```python
from build123d import *

# Parameters (mm, degrees)
BOSS_EXTRUDE1_DEPTH = 12
BOSS_EXTRUDE2_DEPTH = 4.5
FILLET1_R           = 5
FILLET2_R           = 1.5
CUT_EXTRUDE1_DEPTH  = 1
CUT_EXTRUDE2_DEPTH  = 1.5
CUT_EXTRUDE3_DEPTH  = 0.5
FILLET3_R           = 1.5


with BuildPart() as part:
    # Sketch1 → Boss-Extrude1 (new body)
    with BuildSketch(Plane(origin=(0, 0, 0), x_dir=(1, 0, 0), z_dir=(0, 1, 0))):
        with BuildLine():
            Line((-149.337, -110.617), (149.337, -110.617))
            ThreePointArc((149.337, -110.617), (154.286747468, -108.566747468), (156.337, -103.617))
            Line((156.337, -103.617), (156.337, 103.617))
            ThreePointArc((156.337, 103.617), (154.286747468, 108.566747468), (149.337, 110.617))
            Line((149.337, 110.617), (-149.337, 110.617))
            ThreePointArc((-149.337, 110.617), (-154.286747468, 108.566747468), (-156.337, 103.617))
            Line((-156.337, 103.617), (-156.337, -103.617))
            ThreePointArc((-156.337, -103.617), (-154.286747468, -108.566747468), (-149.337, -110.617))
        make_face()
    extrude(amount=BOSS_EXTRUDE1_DEPTH)

    # Sketch2 → Boss-Extrude2 (add)
    with BuildSketch(Plane(origin=(0, 0, -110.617), x_dir=(-1, 0, 0), z_dir=(0, 0, -1))):
        with BuildLine():
            Line((-149.337, 6), (149.337, 6))
            ThreePointArc((149.337, 6), (154.286747468, 8.050252532), (156.337, 13))
            Line((156.337, 13), (156.337, 221))
            ThreePointArc((156.337, 221), (154.286747468, 225.949747468), (149.337, 228))
            Line((149.337, 228), (-149.337, 228))
            ThreePointArc((-149.337, 228), (-154.286747468, 225.949747468), (-156.337, 221))
            Line((-156.337, 221), (-156.337, 13))
            ThreePointArc((-156.337, 13), (-154.286747468, 8.050252532), (-149.337, 6))
        make_face()
    extrude(amount=BOSS_EXTRUDE2_DEPTH)

    # Fillet1
    fillet1_edges = [part.edges().sort_by_distance(p)[0] for p in [
        (-156.337, 0, 0),
        (-154.286747468, 0, -108.566747468),
        (0, 0, -110.617),
        (154.286747468, 0, -108.566747468),
        (156.337, 0, 0),
        (154.286747468, 0, 108.566747468),
        (0, 0, 110.617),
        (-154.286747468, 0, 108.566747468),
    ]]
    fillet(fillet1_edges, radius=FILLET1_R)

    # Fillet2
    fillet2_edges = [part.edges().sort_by_distance(p)[0] for p in [
        (154.286747468, 8.050252532, -115.117),
        (0, 6, -115.117),
        (-154.286747468, 8.050252532, -115.117),
        (-156.337, 117, -115.117),
        (-154.286747468, 225.949747468, -115.117),
        (0, 228, -115.117),
        (154.286747468, 225.949747468, -115.117),
        (156.337, 117, -115.117),
    ]]
    fillet(fillet2_edges, radius=FILLET2_R)

    # Sketch3 → Cut-Extrude1 (cut)
    with BuildSketch(Plane.XY.offset(-110.617)):
        with BuildLine():
            Line((-151.337, 8.417424305), (151.337, 8.417424305))
            ThreePointArc((151.337, 8.417424305), (153.520300133, 10.261387212), (154.337, 13))
            Line((154.337, 13), (154.337, 221))
            ThreePointArc((154.337, 221), (152.872533906, 224.535533906), (149.337, 226))
            Line((149.337, 226), (-149.337, 226))
            ThreePointArc((-149.337, 226), (-152.872533906, 224.535533906), (-154.337, 221))
            Line((-154.337, 221), (-154.337, 13))
            ThreePointArc((-154.337, 13), (-153.520300133, 10.261387212), (-151.337, 8.417424305))
        make_face()
    extrude(amount=-CUT_EXTRUDE1_DEPTH, mode=Mode.SUBTRACT)

    # Sketch4 → Cut-Extrude2 (cut)
    with BuildSketch(Plane(origin=(0, 12, 0), x_dir=(1, 0, 0), z_dir=(0, 1, 0))):
        with BuildLine():
            Line((-134.337, -20.617), (134.337, -20.617))
            ThreePointArc((134.337, -20.617), (137.872533906, -19.152533906), (139.337, -15.617))
            Line((139.337, -15.617), (139.337, 88.617))
            ThreePointArc((139.337, 88.617), (137.872533906, 92.152533906), (134.337, 93.617))
            Line((134.337, 93.617), (-134.337, 93.617))
            ThreePointArc((-134.337, 93.617), (-137.872533906, 92.152533906), (-139.337, 88.617))
            Line((-139.337, 88.617), (-139.337, -15.617))
            ThreePointArc((-139.337, -15.617), (-137.872533906, -19.152533906), (-134.337, -20.617))
        make_face()
    extrude(amount=-CUT_EXTRUDE2_DEPTH, mode=Mode.SUBTRACT)

    # Sketch4<3> → Cut-Extrude3 (cut)
    with BuildSketch(Plane(origin=(0, 12, 0), x_dir=(1, 0, 0), z_dir=(0, 1, 0))):
        with BuildLine():
            Line((-59.837, -23.767), (59.837, -23.767))
            ThreePointArc((59.837, -23.767), (63.372533906, -25.231466094), (64.837, -28.767))
            Line((64.837, -28.767), (64.837, -100.117))
            ThreePointArc((64.837, -100.117), (63.372533906, -103.652533906), (59.837, -105.117))
            Line((59.837, -105.117), (-59.837, -105.117))
            ThreePointArc((-59.837, -105.117), (-63.372533906, -103.652533906), (-64.837, -100.117))
            Line((-64.837, -100.117), (-64.837, -28.767))
            ThreePointArc((-64.837, -28.767), (-63.372533906, -25.231466094), (-59.837, -23.767))
        make_face()
    extrude(amount=-CUT_EXTRUDE3_DEPTH, mode=Mode.SUBTRACT)

    # Fillet3
    fillet3_edges = [part.edges().sort_by_distance(p)[0] for p in [
        (-137.872533906, 10.5, -92.152533906),
        (-139.337, 10.5, -36.5),
        (-137.872533906, 10.5, 19.152533906),
        (0, 10.5, 20.617),
        (137.872533906, 10.5, 19.152533906),
        (139.337, 10.5, -36.5),
        (137.872533906, 10.5, -92.152533906),
        (0, 10.5, -93.617),
    ]]
    fillet(fillet3_edges, radius=FILLET3_R - 0.0001)  # a hair under: the kernel refuses the full size


solid = part.part
```
Geometry check sheet. Reference: the model listing, model coordinates, mm. A direction names the side the tool comes from. Give positions to 0.01 mm unless a question says otherwise; leave off trailing zeros. Write each loop counter-clockwise with the first axis right and the second up, starting at its lowest first coordinate (ties: lowest second). Pieces come first, ordered by that corner, then holes.
1) Material ranges on L1, parallel to Z at x = -51, y = 23.5; L2, parallel to Y at x = -143.5, z = 37; L3, parallel to Y at x = -8.5, z = 86.5, recorded low to high.
2) Section check B-B, the plane y = 203. Record the boundary of the cut face in (x, z), and give its area (3 significant figures).
3) Gauge pin test, flat ends, axial feed: pin 1 (1.5 mm diameter, centred on x = -11.5, y = 67, fed in from +Z); pin 2 (3.5 mm diameter, centred on x = 52.5, z = -112, fed in from -Y). Record the tip position at first contact, or that the pin passes through.
4) Release check for a two-part mould opening along Y. For faces 1 (the cylindrical face through (154.341, 8.105, -112.096)), 2 (the flat face through (2, 119, -115.117)), 3 (the flat face through (-2, 10.5, -37)), 4 (the flat face through (-2, 119, -111.617)) record: pulls with the +Y half, pulls with the -Y half, needs draft (parallel to the pull), parting line crosses it, or undercut.
5) Section check C-C, the plane z = 87. Record the boundary of the cut face in (x, y).
6) Access from +Z, -Z, +X, -X, +Y, -Y to the whole of each face (thin tool, end or side, straight path). Record for faces 5 (the cylindrical face through (-154.232, 7.996, -112.096)), 6 (the flat face through (-2, 12, 23)), 7 (the flat face through (1, 11.5, 64)), 8 (the cylindrical face through (154.232, 8.451, 108.621)), 9 (the cylindrical face through (-154.341, 225.895, -112.096)).
Computed:
1. L1: z = -115.12 to -111.62
1. L2: y = 0 to 12
1. L3: y = 0 to 11.5
2. outline: (-156.34, -113.62) arc R1.5 ccw to (-154.84, -115.12) - (154.84, -115.12) arc R1.5 ccw to (156.34, -113.62) - (156.34, -110.62) - (154.34, -110.62) - (154.34, -111.62) - (-154.34, -111.62) - (-154.34, -110.62) - (-156.34, -110.62) - close
2. area: 1,100 mm2
3. pin 1: stops at z = -111.62
3. pin 2: stops at y = 3.12
4. face 1: pulls with the -Y half
4. face 2: needs draft
4. face 3: pulls with the +Y half
4. face 4: undercut
5. outline: (-156.34, 5) arc R5 ccw to (-151.34, 0) - (151.34, 0) arc R5 ccw to (156.34, 5) - (156.34, 12) - (64.84, 12) - (64.84, 11.5) - (-64.84, 11.5) - (-64.84, 12) - (-156.34, 12) - close
6. face 5: -Z, -X, -Y
6. face 6: +Z, +X, -X, +Y
6. face 7: +Y
6. face 8: +Z, +X, +Y, -Y
6. face 9: +Z, -Z, -X, +Y
